from build123d import *

# Parameters (mm, degrees)
SKETCH2_R           = 37.973
SKETCH2_R_2         = 20.193
BOSS_EXTRUDE1_DEPTH = 3.175
SKETCH4_R           = 1.25
CUT_EXTRUDE1_DEPTH  = 55.07605716


with BuildPart() as part:
    # Sketch2 → Boss-Extrude1 (new, symmetric)
    with BuildSketch(Plane(origin=(0, 0, 0), x_dir=(1, 0, 0), z_dir=(0, 1, 0))):
        with Locations(Location((0, 0, 0), (0, 0, 270))):
            Circle(SKETCH2_R)
        with Locations(Location((0, 0, 0), (0, 0, 270))):
            Circle(SKETCH2_R_2, mode=Mode.SUBTRACT)
    extrude(amount=BOSS_EXTRUDE1_DEPTH, both=True)

    # Sketch4 → Cut-Extrude1 (cut, through all)
    with BuildSketch(Plane(origin=(0, 3.175, 0), x_dir=(1, 0, 0), z_dir=(0, 1, 0))):
        with Locations(Location((-22.987, -13.271550638, 0), (0, 0, 270))):
            Circle(SKETCH4_R)
        with Locations(Location((0, 26.543101276, 0), (0, 0, 270))):
            Circle(SKETCH4_R)
        with Locations(Location((22.987, -13.271550638, 0), (0, 0, 270))):
            Circle(SKETCH4_R)
    extrude(amount=-CUT_EXTRUDE1_DEPTH, mode=Mode.SUBTRACT)


solid = part.part
Design review of the part built by this model. Coordinates are the model's own, in mm. Round coordinates to 2 decimals unless told otherwise and drop trailing zeros. Order: outer loops, then holes, each group sorted by start corner. A loop starts at its lowest first (then second) coordinate and runs counter-clockwise, first axis right, second up. Notation, with made-up numbers: M 44.5,-17.75 L 81.5,-17.75 A26 cw 81.5,-3.75 Z; hole C -6.75,18.25 d6. An arc over 180 degrees is marked long. Answer as CSV lines item,"result". Start each with the question number.
1) Add section B-B (z = 0). Give the boundary of the cut face in (x, y) (3 decimals), then the cut area to 3 significant figures.
2) Wall thickness on line 1 along X through (y, z) = (1, 0); line 2 along X through (y, z) = (1, 12.5); line 3 along X through (y, z) = (-2, -9.5): over which ranges is each line inside the solid? List them lowest first. Write a range as [from, to].
3) The part is to be moulded in two halves that separate along Z. For faces 1 (the face through (-16, -3.175, 16)), 2 (the face through (11.41, 0.04, 36.22)), 3 (the face through (6.07, -0.04, 19.26)), 4 (the face through (-24.207, 0.044, 13.001)), say which applies: +Z half, -Z half, draft (parallel to the pull), parting line (faces both ways), or undercut.
4) Add section D-D (y = 1.75). Give the boundary of the cut face in (x, z), then the cut area to 3 significant figures.
5) Add section A-A (x = 0). Give the boundary of the cut face in (y, z) (3 decimals), then the cut area to 3 significant figures.
6) Add section C-C (x = -12.5). Give the boundary of the cut face in (y, z) (3 decimals).
7) For pin 1 Ø2 at (x, y) = (-11.5, -0.5) entering from +Z; pin 2 Ø1.5 at (y, z) = (-1, -27) entering from +X; pin 3 Ø2 at (x, y) = (28, -2) entering from -Z, all flat-tipped, find the tip position at first contact; note any pin that passes through.
Resolved:
1,outline,"M -37.973,-3.175 L -20.193,-3.175 L -20.193,3.175 L -37.973,3.175 Z; M 20.193,-3.175 L 37.973,-3.175 L 37.973,3.175 L 20.193,3.175 Z"
1,area,"226 mm^2"
2,line 1,"[-37.97, -20.19], [20.19, 37.97]"
2,line 2,"[-35.86, -23.97], [-22, -15.86], [15.86, 22], [23.97, 35.86]"
2,line 3,"[-36.77, -17.82], [17.82, 36.77]"
3,face 1,"draft"
3,face 2,"parting line"
3,face 3,"undercut"
3,face 4,"undercut"
4,outline,"C 0,0 d75.95; hole C -22.99,13.27 d2.5; hole C 0,0 d40.39; hole C 0,-26.54 d2.5; hole C 22.99,13.27 d2.5"
4,area,"3,230 mm^2"
5,outline,"M -3.175,-37.973 L 3.175,-37.973 L 3.175,-27.793 L -3.175,-27.793 Z; M -3.175,-25.293 L 3.175,-25.293 L 3.175,-20.193 L -3.175,-20.193 Z; M -3.175,20.193 L 3.175,20.193 L 3.175,37.973 L -3.175,37.973 Z"
5,area,"210 mm^2"
6,outline,"M -3.175,-35.857 L 3.175,-35.857 L 3.175,-15.859 L -3.175,-15.859 Z; M -3.175,15.859 L 3.175,15.859 L 3.175,35.857 L -3.175,35.857 Z"
7,pin 1,"z = 36.49"
7,pin 2,"x = 27.44"
7,pin 3,"z = -26.7"
